The listing builds one solid part. Answer for the finished solid, in the listing's coordinates (mm). A direction names the side the tool comes from. Coordinates: 2 decimals unless noted, no trailing zeros. Write each loop counter-clockwise with the first axis right and the second up, starting at its lowest first coordinate (ties: lowest second). Pieces come first, ordered by that corner, then holes.
(1) The part is cut by section A-A on x = 99. Determine the outline of the cut face in (y, z), plus the area to 3 significant figures.
(2) The part is cut by section D-D on z = -20. Determine the outline of the cut face in (x, y).
(3) A straight line is drawn through the part: line 1 (X direction, y = 14.75, z = -22.5). Find the intervals that lie inside material, in ascending order.
(4) Which of the six approach directions +Z, -Z, +X, -X, +Y, -Y give full straight-line access (tool end or side, diameter ignored) to faces 5 (the flat face through (100, 18, -17)), 6 (the flat face through (52, 26, -27)), 7 (the flat face through (87, 10, -5))?
(5) The part is cut by section C-C on z = -3.5. Determine the outline of the cut face in (x, y), plus the area to 3 significant figures.
(6) For a pull along X with two mould halves and no side action, classify faces 1 (the flat face through (52, 13, 0)), 2 (the flat face through (95, 16, -17)), 3 (the flat face through (87, 7, -2)), 4 (the flat face through (80, 10, -2)) as +X half, -X half, draft (parallel to the pull), parting line (faces both ways), or undercut.
(7) Given P1, Ø1.5, axis at y = 14.5, z = -14.5, coming from the +X side; P2, Ø1.8, axis at x = 87, y = 11, coming from the +Z side, each flat-ended and moving along its own axis, determine where each tip first touches the part or whether it passes through.
(8) The part is cut by section B-B on y = 14.25. Determine the outline of the cut face in (x, z).
from build123d import *

# Parameters (mm, degrees)
SKETCH2_W           = 105
SKETCH2_H           = 53
BOSS_EXTRUDE1_DEPTH = 26
SKETCH3_W           = 15
SKETCH3_H           = 6
CUT_EXTRUDE1_DEPTH  = 5
SKETCH4_W           = 15
SKETCH4_H           = 5
CUT_EXTRUDE2_DEPTH  = 10


with BuildPart() as part:
    # Sketch2 → Boss-Extrude1 (new body)
    with BuildSketch(Plane(origin=(0, 0, 0), x_dir=(1, 0, 0), z_dir=(0, 1, 0))):
        with Locations((52.5, 26.5)):
            Rectangle(SKETCH2_W, SKETCH2_H)
    extrude(amount=BOSS_EXTRUDE1_DEPTH)

    # Sketch3 → Cut-Extrude1 (cut)
    with BuildSketch(Plane.XY):
        with Locations((87.5, 10)):
            Rectangle(SKETCH3_W, SKETCH3_H)
    extrude(amount=-CUT_EXTRUDE1_DEPTH, mode=Mode.SUBTRACT)

    # Sketch4 → Cut-Extrude2 (cut)
    with BuildSketch(Plane(origin=(105, 0, 0), x_dir=(0, 0, -1), z_dir=(1, 0, 0))):
        with Locations((17.5, 15.5)):
            Rectangle(SKETCH4_W, SKETCH4_H)
    extrude(amount=-CUT_EXTRUDE2_DEPTH, mode=Mode.SUBTRACT)


solid = part.part
Model answer:
1. outline: (0, -53) - (26, -53) - (26, 0) - (0, 0) - close; hole (13, -25) - (18, -25) - (18, -10) - (13, -10) - close
1. area: 1,300 mm2
2. outline: (0, 0) - (105, 0) - (105, 13) - (95, 13) - (95, 18) - (105, 18) - (105, 26) - (0, 26) - close
3. line 1: x = 0 to 95
4. face 5: +X
4. face 6: +Z, -Z, +X, -X, +Y
4. face 7: +Z
5. outline: (0, 0) - (105, 0) - (105, 26) - (0, 26) - close; hole (80, 7) - (95, 7) - (95, 13) - (80, 13) - close
5. area: 2,640 mm2
6. face 1: draft
6. face 2: +X half
6. face 3: undercut
6. face 4: undercut
7. P1: stops at x = 95
7. P2: stops at z = -5
8. outline: (0, -53) - (105, -53) - (105, -25) - (95, -25) - (95, -10) - (105, -10) - (105, 0) - (0, 0) - close
